Source: CAD feature listing. Evaluate the final solid. Frame: model axes, mm. Coordinates: 2 decimals unless noted, no trailing zeros. Order: outer loops, then holes, each group sorted by start corner. A loop starts at its lowest first (then second) coordinate and runs counter-clockwise, first axis right, second up. Notation, with made-up numbers: (77, 3.5) -> (83, 3.5) arc R33 ccw to (83, 33.5) -> close; hole circle Ø2 at (-38.75, 38). An arc over 180 degrees is marked (long way). Put each result on its own line as item: value.
from build123d import *

# Parameters (mm, degrees)
F0_W     = 100
F0_H     = 40
F1_DEPTH = 6
F2_R     = 3.5
F3_DEPTH = 6.001


with BuildPart() as f1:
    # F0 (on Front) → F1 (new body)
    with BuildSketch(Plane.XZ):
        with Locations((50, 20)):
            Rectangle(F0_W, F0_H)
        Polygon((100, 0), (0, 0), (20, -20), (80, -20), align=None)
    extrude(amount=F1_DEPTH)

    # F2 (on face) → F3 (cut, through all)
    with BuildSketch(Plane.XZ.offset(6)):
        with Locations((8, 26)):
            Circle(F2_R)
        with Locations((92, 26)):
            Circle(F2_R)
    extrude(amount=-F3_DEPTH, mode=Mode.SUBTRACT)


solid = f1.part
1. First-contact query: pin 1 (3 mm diameter, centred on y = -2, z = -11, fed in from -X). Flat tip, straight axial feed; report the tip coordinate or a pass-through.
Numbers:
pin 1: stops at x = 9.5
2. Cut plane C-C on y = -2.65. Output: boundary loops of the cut face in (x, z), plus the area to 3 significant figures.
Numbers:
outline: (0, 0) -> (20, -20) -> (80, -20) -> (100, 0) -> (100, 40) -> (0, 40) -> close; hole circle Ø7 at (8, 26); hole circle Ø7 at (92, 26)
area: 5,520 mm2
3. Ray query, line 1 along Z through (x, y) = (8, -4.1); line 2 along X through (y, z) = (-3.05, -2.5); line 3 along X through (y, z) = (-3.85, -16). Return the intervals inside material, ascending.
Numbers:
line 1: z = -8 to 22.5, 29.5 to 40
line 2: x = 2.5 to 97.5
line 3: x = 16 to 84
4. Cut plane A-A on x = 8. Output: boundary loops of the cut face in (y, z), plus the area to 3 significant figures.
Numbers:
outline: (-6, -8) -> (0, -8) -> (0, 22.5) -> (-6, 22.5) -> close; (-6, 29.5) -> (0, 29.5) -> (0, 40) -> (-6, 40) -> close
area: 246 mm2
5. Cut plane D-D on z = -4.5. Output: boundary loops of the cut face in (x, y).
Numbers:
outline: (4.5, -6) -> (95.5, -6) -> (95.5, 0) -> (4.5, 0) -> close
6. Cut plane B-B on z = 26. Output: boundary loops of the cut face in (x, y).
Numbers:
outline: (0, -6) -> (4.5, -6) -> (4.5, 0) -> (0, 0) -> close; (11.5, -6) -> (88.5, -6) -> (88.5, 0) -> (11.5, 0) -> close; (95.5, -6) -> (100, -6) -> (100, 0) -> (95.5, 0) -> close
7. Pull-direction query (Z, two-part tool) for faces 1 (the flat face through (10, -3, -10)), 2 (the flat face through (49, -3, 40)), 3 (the cylindrical face through (5.42, -3.042, 28.365)); classes: pulls with the +Z half, pulls with the -Z half, needs draft (parallel to the pull), parting line crosses it, or undercut.
Numbers:
face 1: pulls with the -Z half
face 2: pulls with the +Z half
face 3: undercut
